Part model, mm, in its own coordinate system. Face numbers are marked on the shaded views. Coordinates: 2 decimals unless noted, no trailing zeros. Order: outer loops, then holes, each group sorted by start corner. A loop starts at its lowest first (then second) coordinate and runs counter-clockwise, first axis right, second up.
1) Cut at A-A (z = 0). List the corners of the cut face in (x, y).
2) Mould opens along X. For the marked faces 1 and 2 say: +X half, -X half, draft (parallel to the pull), parting line (faces both ways), or undercut.
3) Wall check: L1, parallel to X at y = 1.35, z = 0; L2, parallel to Z at x = 0, y = 0.8; L3, parallel to X at y = 1.1, z = 9. Give the ranges that are in metal, low to high.
4) Pin check, flat tips, straight feed: pin 1 Ø9 at (x, z) = (0, 0) entering from -Y; pin 2 Ø1 at (y, z) = (1, 10.5) entering from +X; pin 3 Ø0.5 at (x, y) = (0, 2.5) entering from -Z. Stop position of each tip, or through.
```python
from build123d import *

# Parameters (mm, degrees)
SKETCH1_R           = 34.5
BOSS_EXTRUDE1_DEPTH = 4
CUT_EXTRUDE1_DEPTH  = 4
SKETCH3_R           = 32.5
SKETCH3_R_2         = 12.5
SKETCH3_R_3         = 7.5
CUT_EXTRUDE2_DEPTH  = 2
SKETCH4_W           = 5.931596908
SKETCH4_H           = 30.157362647
CUT_EXTRUDE3_DEPTH  = 2
FILLET1_R           = 1


with BuildPart() as part:
    # Sketch1 → Boss-Extrude1 (new body)
    with BuildSketch(Plane(origin=(0, 0, 0), x_dir=(1, 0, 0), z_dir=(0, 1, 0))):
        Circle(SKETCH1_R)
    extrude(amount=BOSS_EXTRUDE1_DEPTH)

    # Sketch2 → Cut-Extrude1 (cut)
    with BuildSketch(Plane(origin=(0, 4, 0), x_dir=(1, 0, 0), z_dir=(0, 1, 0))):
        with BuildLine():
            Line((0.5, -2.5), (-0.5, -2.5))
            ThreePointArc((-0.5, -2.5), (-3, 0), (-0.5, 2.5))
            Line((-0.5, 2.5), (0.5, 2.5))
            ThreePointArc((0.5, 2.5), (3, 0), (0.5, -2.5))
        make_face()
    extrude(amount=-CUT_EXTRUDE1_DEPTH, mode=Mode.SUBTRACT)

    # Sketch3 → Cut-Extrude2 (cut)
    with BuildSketch(Plane.XZ):
        Circle(SKETCH3_R)
        Circle(SKETCH3_R_2, mode=Mode.SUBTRACT)
        Circle(SKETCH3_R_3)
        with BuildLine():
            ThreePointArc((-0.5, -2.5), (-3, 0), (-0.5, 2.5))
            Line((-0.5, 2.5), (0.5, 2.5))
            ThreePointArc((0.5, 2.5), (3, 0), (0.5, -2.5))
            Line((0.5, -2.5), (-0.5, -2.5))
        make_face(mode=Mode.SUBTRACT)
    extrude(amount=-CUT_EXTRUDE2_DEPTH, mode=Mode.SUBTRACT)

    # Sketch4 → Cut-Extrude3 (cut)
    with BuildSketch(Plane.XZ):
        with Locations((0, 21.96737057)):
            Rectangle(SKETCH4_W, SKETCH4_H)
    extrude(amount=-CUT_EXTRUDE3_DEPTH, mode=Mode.SUBTRACT)

    # Fillet1
    fillet1_edges = [part.edges().sort_by_distance(p)[0] for p in [
        (-23.323056761, 0, -25.422136482),
    ]]
    fillet(fillet1_edges, radius=FILLET1_R)


solid = part.part
```
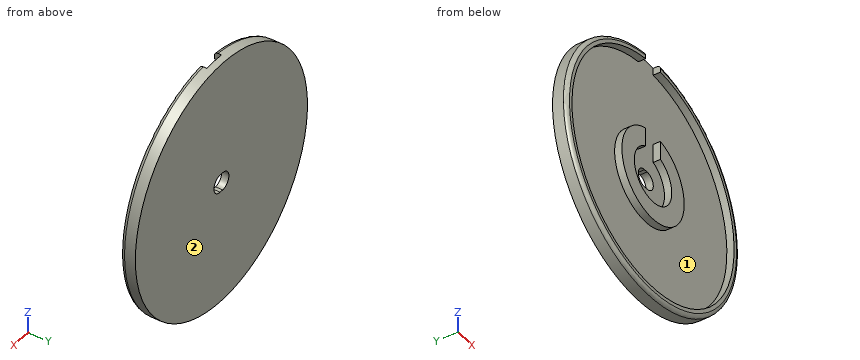
Geometry check:
1. outline: (-34.5, 1) arc R1 ccw to (-33.5, 0) - (-32.5, 0) - (-32.5, 2) - (-12.5, 2) - (-12.5, 0) - (-7.5, 0) - (-7.5, 2) - (-3, 2) - (-3, 4) - (-34.5, 4) - close; (3, 2) - (7.5, 2) - (7.5, 0) - (12.5, 0) - (12.5, 2) - (32.5, 2) - (32.5, 0) - (33.5, 0) arc R1 ccw to (34.5, 1) - (34.5, 4) - (3, 4) - close
2. face 1: undercut
2. face 2: draft
3. L1: x = -34.5 to -32.5, -12.5 to -7.5, 7.5 to 12.5, 32.5 to 34.5
3. L2: z = -34.48 to -32.5, -12.5 to -7.5
3. L3: x = -33.31 to -31.23, -8.67 to -2.97, 2.97 to 8.67, 31.23 to 33.31
4. pin 1: stops at y = 2
4. pin 2: stops at x = 33.02
4. pin 3: stops at z = -34.5
